Could you check a few things on this model? Use its own coordinates, in mm. A direction names the side the tool comes from. Round coordinates to 2 decimals unless told otherwise and drop trailing zeros. Loops run counter-clockwise (first coordinate to the right, second up) from the corner with the lowest first, then second, coordinate; pieces in that order, holes last. Notation, with made-up numbers: (-39.75, 17) -> (2.25, 17) arc R20 ccw to (2.25, 48) -> close; hole circle Ø3 at (81, 65.5). An arc over 180 degrees is marked (long way). Write each question's results on one line, items separated by ' | '. Start each with the question number.
1) Imagine slicing it at A-A, the plane z = 0. List the corners of the cut face in (x, y) for me (1 decimal), plus the area to 3 significant figures.
2) If I drill on probe 1 along Z at (x, y) = (14, -27); probe 2 along Y at (x, z) = (0, 16.4); probe 3 along Z at (x, y) = (15.5, -0.5), over which ranges is the centre line in solid material (lowest first)?
3) Which directions (+Z, -Z, +X, -X, +Y, -Y) give clear straight access to the entire face, cutting with the end or side of a thin tool? Please do faces 1 (the flat face through (0, -26, 16.5)), 2 (the flat face through (0, -30.828, -14)), 3 (the flat face through (10, 11, 14.288)), 4 (the flat face through (0, -29, 13.5)), 5 (the cylindrical face through (-1.82, 13.85, 16.72)).
4) Imagine slicing it at D-D, the plane x = -20.5. List the corners of the cut face in (y, z) for me.
5) Imagine slicing it at B-B, the plane x = 0. List the corners of the cut face in (y, z) for me, plus the area to 3 significant figures.
6) For P1, Ø4, axis at x = -35.5, z = -0.5, coming from the +Y side; P2, Ø4, axis at y = -7, z = 15.5, coming from the +X side (3 decimals); P3, Ø3.5, axis at y = -29.5, z = -4.5, coming from the -X side; P4, Ø2, axis at x = 33.89, y = 11.44, coming from the +Z side, each with a flat end and sliding along its axis, tell me the tip position at first contact or that it passes through.
7) We'd pull the mould along Z, two halves only. Please class faces 6 (the flat face through (34, 14, -19.964)), 7 (the flat face through (21, -24, 8)), 8 (the flat face through (21, -26.828, 0)), 9 (the flat face through (-32, -10.828, -16)): pulls with the +Z half, pulls with the -Z half, needs draft (parallel to the pull), parting line crosses it, or undercut.
8) Imagine slicing it at C-C, the plane y = 0. List the corners of the cut face in (x, z) for me (1 decimal), plus the area to 3 significant figures.
from build123d import *

# Parameters (mm, degrees)
SKETCH1_W                 = 36.575
SKETCH1_H                 = 41.655
SKETCH1_W_2               = 28.575
SKETCH1_H_2               = 33.655
BOSS_EXTRUDE1_DEPTH       = 41.275
SKETCH2_W                 = 36.575
SKETCH2_H                 = 41.655
BOSS_EXTRUDE2_DEPTH       = 2
SKETCH3_W                 = 86.55
SKETCH3_H                 = 36.575
CUT_EXTRUDE1_DEPTH        = 4
SKETCH4_W                 = 10.7752
SKETCH4_H                 = 10.7752
SKETCH4_W_2               = 4.7752
SKETCH4_H_2               = 4.7752
BOSS_EXTRUDE3_DEPTH       = 1.6764
MIRROR3_COPY_1_SKETCH_W   = 10.7752
MIRROR3_COPY_1_SKETCH_H   = 10.7752
MIRROR3_COPY_1_SKETCH_W_2 = 4.7752
MIRROR3_COPY_1_SKETCH_H_2 = 4.7752
MIRROR3_COPY_1_DEPTH      = 1.6764
SKETCH5_R                 = 1.1
CUT_EXTRUDE2_DEPTH        = 62.397719691
SKETCH6_R                 = 4
BOSS_EXTRUDE4_DEPTH       = 6
SKETCH7_R                 = 12.7
CUT_EXTRUDE3_DEPTH        = 4
SKETCH8_R                 = 13.97
CUT_EXTRUDE4_DEPTH        = 3.175
SKETCH9_W                 = 14.4
SKETCH9_H                 = 6
CUT_EXTRUDE5_DEPTH        = 4
SKETCH10_W                = 45
SKETCH10_H                = 33
SKETCH10_W_2              = 37
SKETCH10_H_2              = 25
BOSS_EXTRUDE5_DEPTH       = 10
SKETCH11_W                = 39
SKETCH11_H                = 27
CUT_EXTRUDE7_DEPTH        = 3.175
SKETCH14_W                = 16
SKETCH14_H                = 6
CUT_EXTRUDE8_DEPTH        = 4


with BuildPart() as part:
    # Sketch1 → Boss-Extrude1 (new, symmetric)
    with BuildSketch(Plane(origin=(0, 0, 0), x_dir=(0, 0, -1), z_dir=(1, 0, 0))):
        Rectangle(SKETCH1_W, SKETCH1_H)
        Rectangle(SKETCH1_W_2, SKETCH1_H_2, mode=Mode.SUBTRACT)
    extrude(amount=BOSS_EXTRUDE1_DEPTH, both=True)

    # Sketch2 → Boss-Extrude2 (add)
    with BuildSketch(Plane.ZY.offset(41.275)):
        Rectangle(SKETCH2_W, SKETCH2_H)
    boss_extrude2 = extrude(amount=BOSS_EXTRUDE2_DEPTH)

    # Mirror1: Boss-Extrude2 across plane
    add(boss_extrude2.mirror(Plane(origin=(0, 0, 0), x_dir=(0, 0, 1), z_dir=(1, 0, 0))))

    # Sketch3 → Cut-Extrude1 (cut)
    with BuildSketch(Plane(origin=(0, 20.8275, 0), x_dir=(1, 0, 0), z_dir=(0, 1, 0))):
        Rectangle(SKETCH3_W, SKETCH3_H)
    extrude(amount=-CUT_EXTRUDE1_DEPTH, mode=Mode.SUBTRACT)

    # Sketch4 → Boss-Extrude3 (add)
    with BuildSketch(Plane(origin=(0, 0, -18.2875), x_dir=(-1, 0, 0), z_dir=(0, 0, -1))):
        with Locations((-33.8874, 11.4399)):
            Rectangle(SKETCH4_W, SKETCH4_H)
        with Locations((-33.8874, 11.4399)):
            Rectangle(SKETCH4_W_2, SKETCH4_H_2, mode=Mode.SUBTRACT)
    boss_extrude3 = extrude(amount=BOSS_EXTRUDE3_DEPTH)

    # Mirror2: Boss-Extrude3 across plane
    add(boss_extrude3.mirror(Plane(origin=(0, 0, 0), x_dir=(0, 0, 1), z_dir=(1, 0, 0))))

    # Mirror3: Boss-Extrude3 across plane
    add(boss_extrude3.mirror(Plane.XY))

    # Mirror3 copy 1 sketch → Mirror3 copy 1 (add)
    with BuildSketch(Plane.XY.offset(18.2875)):
        with Locations((-33.8874, 11.4399)):
            Rectangle(MIRROR3_COPY_1_SKETCH_W, MIRROR3_COPY_1_SKETCH_H)
        with Locations((-33.8874, 11.4399)):
            Rectangle(MIRROR3_COPY_1_SKETCH_W_2, MIRROR3_COPY_1_SKETCH_H_2, mode=Mode.SUBTRACT)
    extrude(amount=MIRROR3_COPY_1_DEPTH)

    # Sketch5 → Cut-Extrude2 (cut, through all)
    with BuildSketch(Plane.XY.offset(18.2875)):
        with Locations((-33.8874, 11.4399)):
            Circle(SKETCH5_R)
    cut_extrude2 = extrude(amount=-CUT_EXTRUDE2_DEPTH, mode=Mode.SUBTRACT)

    # Mirror4: Cut-Extrude2 across plane
    add(cut_extrude2.mirror(Plane(origin=(0, 0, 0), x_dir=(0, 0, 1), z_dir=(1, 0, 0))), mode=Mode.SUBTRACT)

    # Sketch6 → Boss-Extrude4 (add)
    with BuildSketch(Plane.ZY.offset(43.275)):
        Circle(SKETCH6_R)
    boss_extrude4 = extrude(amount=BOSS_EXTRUDE4_DEPTH)

    # Mirror5: Boss-Extrude4 across plane
    add(boss_extrude4.mirror(Plane(origin=(0, 0, 0), x_dir=(0, 0, 1), z_dir=(1, 0, 0))))

    # Sketch7 → Cut-Extrude3 (cut)
    with BuildSketch(Plane.XY.offset(18.2875)):
        Circle(SKETCH7_R)
    extrude(amount=-CUT_EXTRUDE3_DEPTH, mode=Mode.SUBTRACT)

    # Sketch8 → Cut-Extrude4 (cut)
    with BuildSketch(Plane.XY.offset(18.2875)):
        Circle(SKETCH8_R)
    extrude(amount=-CUT_EXTRUDE4_DEPTH, mode=Mode.SUBTRACT)

    # Sketch9 → Cut-Extrude5 (cut)
    with BuildSketch(Plane(origin=(0, 0, -18.2875), x_dir=(-1, 0, 0), z_dir=(0, 0, -1))):
        with Locations((32.075, -13.8275)):
            Rectangle(SKETCH9_W, SKETCH9_H)
    extrude(amount=-CUT_EXTRUDE5_DEPTH, mode=Mode.SUBTRACT)

    # Sketch10 → Boss-Extrude5 (add)
    with BuildSketch(Plane.XZ.offset(20.8275)):
        Rectangle(SKETCH10_W, SKETCH10_H)
        Rectangle(SKETCH10_W_2, SKETCH10_H_2, mode=Mode.SUBTRACT)
    extrude(amount=BOSS_EXTRUDE5_DEPTH)

    # Sketch11 → Cut-Extrude7 (cut)
    with BuildSketch(Plane.XZ.offset(30.8275)):
        Rectangle(SKETCH11_W, SKETCH11_H)
    extrude(amount=-CUT_EXTRUDE7_DEPTH, mode=Mode.SUBTRACT)

    # Sketch14 → Cut-Extrude8 (cut)
    with BuildSketch(Plane(origin=(22.5, 0, 0), x_dir=(0, 0, -1), z_dir=(1, 0, 0))):
        with Locations((0, -23.8275)):
            Rectangle(SKETCH14_W, SKETCH14_H)
    extrude(amount=-CUT_EXTRUDE8_DEPTH, mode=Mode.SUBTRACT)


solid = part.part
Checked values:
1) outline: (-49.3, -4) -> (-43.3, -4) -> (-43.3, -20.8) -> (-22.5, -20.8) -> (-22.5, -30.8) -> (-19.5, -30.8) -> (-19.5, -27.7) -> (-18.5, -27.7) -> (-18.5, -20.8) -> (43.3, -20.8) -> (43.3, -4) -> (49.3, -4) -> (49.3, 4) -> (43.3, 4) -> (43.3, 16.8) -> (41.3, 16.8) -> (41.3, -16.8) -> (-41.3, -16.8) -> (-41.3, 16.8) -> (-43.3, 16.8) -> (-43.3, 4) -> (-49.3, 4) -> close; (18.5, -27.7) -> (19.5, -27.7) -> (19.5, -30.8) -> (22.5, -30.8) -> (22.5, -26.8) -> (18.5, -26.8) -> close | area: 626 mm^2
2) probe 1: -16.5 to -12.5, 12.5 to 16.5 | probe 2: -30.83 to -13.97, 13.97 to 16.83 | probe 3: -18.29 to -14.29, 14.29 to 18.29
3) face 1: +Z, +X, -X, -Y | face 2: +Z, -Z, +X, -X, -Y | face 3: +Y | face 4: -Y | face 5: +Z
4) outline: (-30.83, -16.5) -> (-20.83, -16.5) -> (-20.83, -18.29) -> (16.83, -18.29) -> (16.83, -14.29) -> (-16.83, -14.29) -> (-16.83, 14.29) -> (16.83, 14.29) -> (16.83, 18.29) -> (-20.83, 18.29) -> (-20.83, 16.5) -> (-30.83, 16.5) -> close
5) outline: (-30.83, -16.5) -> (-20.83, -16.5) -> (-20.83, -18.29) -> (16.83, -18.29) -> (16.83, -14.29) -> (-16.83, -14.29) -> (-16.83, 14.29) -> (-12.7, 14.29) -> (-12.7, 15.11) -> (-13.97, 15.11) -> (-13.97, 18.29) -> (-20.83, 18.29) -> (-20.83, 16.5) -> (-30.83, 16.5) -> (-30.83, 13.5) -> (-27.65, 13.5) -> (-27.65, 12.5) -> (-20.83, 12.5) -> (-20.83, -12.5) -> (-27.65, -12.5) -> (-27.65, -13.5) -> (-30.83, -13.5) -> close; (12.7, 14.29) -> (16.83, 14.29) -> (16.83, 18.29) -> (13.97, 18.29) -> (13.97, 15.11) -> (12.7, 15.11) -> close | area: 380 mm^2
6) P1: y = -16.83 | P2: x = 43.275 | P3: x = -22.5 | P4: through
7) face 6: pulls with the -Z half | face 7: undercut | face 8: undercut | face 9: needs draft
8) outline: (-49.3, -4) -> (-43.3, -4) -> (-43.3, -18.3) -> (43.3, -18.3) -> (43.3, -4) -> (49.3, -4) -> (49.3, 4) -> (43.3, 4) -> (43.3, 18.3) -> (14, 18.3) -> (14, 15.1) -> (12.7, 15.1) -> (12.7, 14.3) -> (41.3, 14.3) -> (41.3, -14.3) -> (-41.3, -14.3) -> (-41.3, 14.3) -> (-12.7, 14.3) -> (-12.7, 15.1) -> (-14, 15.1) -> (-14, 18.3) -> (-43.3, 18.3) -> (-43.3, 4) -> (-49.3, 4) -> close | area: 793 mm^2
